from build123d import *

# Parameters (mm, degrees)
SKETCH1_R           = 11.43
SKETCH1_W           = 6.35
SKETCH1_H           = 6.35
BOSS_EXTRUDE1_DEPTH = 6.35


with BuildPart() as part:
    # Sketch1 → Boss-Extrude1 (new body)
    with BuildSketch(Plane(origin=(0, 0, 0), x_dir=(0, 0, -1), z_dir=(1, 0, 0))):
        Circle(SKETCH1_R)
        with Locations((-6.35, 0)):
            Rectangle(SKETCH1_W, SKETCH1_H, mode=Mode.SUBTRACT)
        with Locations((6.35, 0)):
            Rectangle(SKETCH1_W, SKETCH1_H, mode=Mode.SUBTRACT)
    extrude(amount=BOSS_EXTRUDE1_DEPTH)


solid = part.part
Verification items for the finished model (mm, model axes). A direction names the side the tool comes from. Give positions to 0.01 mm unless a question says otherwise; leave off trailing zeros. Write each loop counter-clockwise with the first axis right and the second up, starting at its lowest first coordinate (ties: lowest second). Pieces come first, ordered by that corner, then holes. Notation, with made-up numbers: M 21,-37.75 L 58,-37.75 A16 ccw 58,-31.75 Z; hole C -35,7.25 d5. An arc over 180 degrees is marked long. Write item = value, one per line.
(1) Sectioned sample at C-C (z = 7.25). Record the cut outline in (x, y) (3 decimals).
Found:
outline = M 0,-8.836 L 6.35,-8.836 L 6.35,-3.175 L 0,-3.175 Z; M 0,3.175 L 6.35,3.175 L 6.35,8.836 L 0,8.836 Z
(2) Sectioned sample at A-A (y = 0). Record the cut outline in (x, z) (3 decimals), then the cut area to 3 significant figures.
Found:
outline = M 0,-11.43 L 6.35,-11.43 L 6.35,-9.525 L 0,-9.525 Z; M 0,-3.175 L 6.35,-3.175 L 6.35,3.175 L 0,3.175 Z; M 0,9.525 L 6.35,9.525 L 6.35,11.43 L 0,11.43 Z
area = 64.5 mm2
(3) Draft check along Z on faces 1 (the face through (3, 0, -9.525)), 2 (the face through (3.131, 3.433, -10.902)), 3 (the face through (0, 0, 0)), 4 (the face through (3, 3.175, 6)). Enter one of: released by +Z, released by -Z, zero draft, split by the parting line, or undercut.
Found:
face_1 = undercut
face_2 = split by the parting line
face_3 = zero draft
face_4 = undercut
(4) Access from +Z, -Z, +X, -X, +Y, -Y to the whole of each face (thin tool, end or side, straight path). Record for faces 5 (the face through (3, 0, 9.525)), 6 (the face through (6.35, 0, 0)).
Found:
face_5 = +X, -X
face_6 = +Z, -Z, +X, +Y, -Y
(5) Sectioned sample at B-B (x = 1.5). Record the cut outline in (y, z) (3 decimals).
Found:
outline = C 0,0 d22.86; hole M -3.175,-9.525 L 3.175,-9.525 L 3.175,-3.175 L -3.175,-3.175 Z; hole M -3.175,3.175 L 3.175,3.175 L 3.175,9.525 L -3.175,9.525 Z
(6) Go/stop test with flat-tipped pins: pin 1 Ø2 at (y, z) = (-7, 8) entering from -X; pin 2 Ø1.9 at (x, z) = (2, -6) entering from +Y; pin 3 Ø1.5 at (x, z) = (2, -5) entering from -Y; pin 4 Ø2 at (y, z) = (0.5, 8) entering from -X. Record where each tip stops, or that it passes through.
Found:
pin_1 = 0
pin_2 = 10.25
pin_3 = -10.61
pin_4 = through
(7) Sectioned sample at D-D (y = 7.75). Record the cut outline in (x, z).
Found:
outline = M 0,-8.4 L 6.35,-8.4 L 6.35,8.4 L 0,8.4 Z
(8) Material ranges on line 1 (Z direction, x = 3, y = -2.5) (3 decimals); line 2 (Z direction, x = 2, y = 2.75) (3 decimals); line 3 (Y direction, x = 6, z = 5.75) (3 decimals), recorded low to high.
Found:
line_1 = -11.153 to -9.525, -3.175 to 3.175, 9.525 to 11.153
line_2 = -11.094 to -9.525, -3.175 to 3.175, 9.525 to 11.094
line_3 = -9.878 to -3.175, 3.175 to 9.878
